Answer from the drawing. Dimensions are ordinates in mm from the lowest x, y and z of the part. Round coordinates to 2 decimals unless told otherwise and drop trailing zeros. Order: outer loops, then holes, each group sorted by start corner. A loop starts at its lowest first (then second) coordinate and runs counter-clockwise, first axis right, second up. Notation, with made-up numbers: M -38,49 L 3,49 A23 ccw 3,63 Z; hole C -6,23 d6. An arc over 180 degrees is marked long. Use one line per item in the form item = value. Start each with the question number.
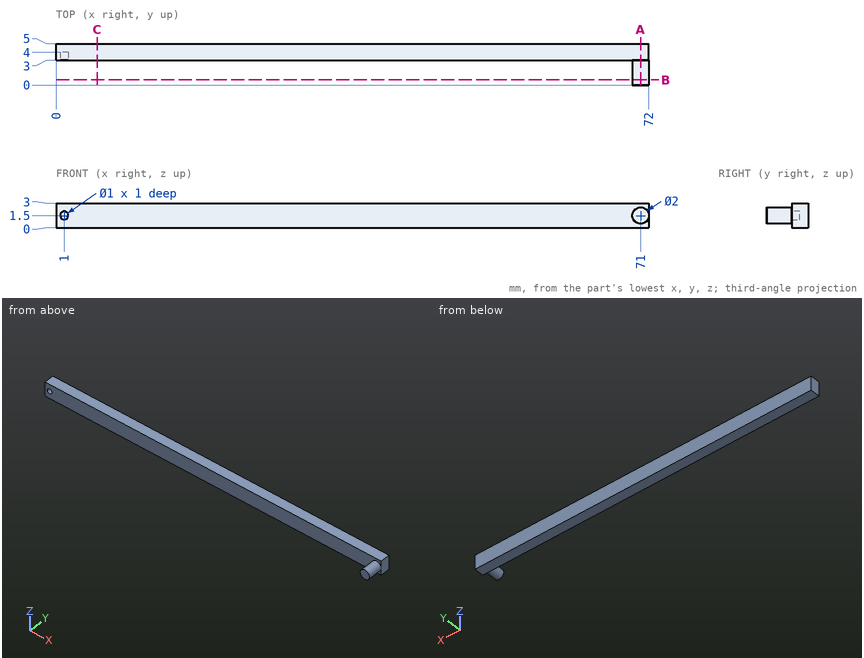
Item 1: Section C-C (x = 5) is taken. Write down the section's boundary in (y, z).
Item 2: Section A-A (x = 71) is taken. Write down the section's boundary in (y, z).
Item 3: Given P1, Ø1, axis at x = 62.5, z = 0.5, coming from the -Y side; P2, Ø0.5, axis at x = 1, z = 1.5, coming from the -Y side; P3, Ø3, axis at x = 50.5, y = 3.5, coming from the -Z side; P4, Ø2, axis at x = 52, y = 0.5, coming from the -Z side, each flat-ended and moving along its own axis, determine where each tip first touches the part or whether it passes through.
Item 4: Find the intervals of material crossed by L1, parallel to X at y = 3.3, z = 1.5; L2, parallel to Z at x = 1, y = 3.5; L3, parallel to Y at x = 26.5, z = 2.35, in increasing order. Write a range as [from, to].
Item 5: Section B-B (y = 0.65) is taken. Write down the section's boundary in (x, z).
The answers:
q1.outline = M 3,0 L 5,0 L 5,3 L 3,3 Z
q2.outline = M 0,0.5 L 3,0.5 L 3,0 L 5,0 L 5,3 L 3,3 L 3,2.5 L 0,2.5 Z
q3.P1 = 3
q3.P2 = 4
q3.P3 = 0
q3.P4 = through
q4.L1 = [0, 0.5], [1.5, 72]
q4.L2 = [0, 1], [2, 3]
q4.L3 = [3, 5]
q5.outline = C 71,1.5 d2
